Here's the drawing with two shaded views (mm, measured from the low corner). I have some questions. A direction names the side the tool comes from. Round coordinates to 2 decimals unless told otherwise and drop trailing zeros. Loops run counter-clockwise (first coordinate to the right, second up) from the corner with the lowest first, then second, coordinate; pieces in that order, holes last.
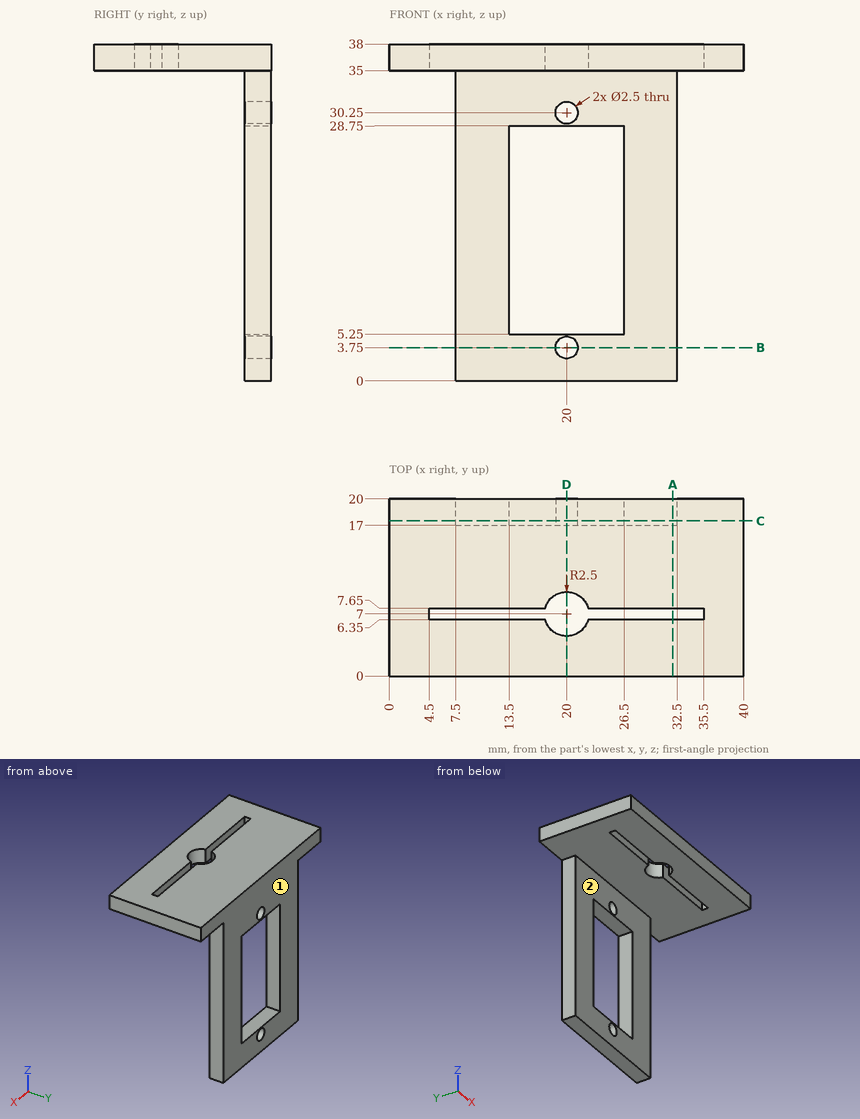
Item 1: If we section it at A-A, the plane x = 32: Please give me the cut outline in (y, z).
Results list:
outline: (0, 35) - (6.35, 35) - (6.35, 38) - (0, 38) - close; (7.65, 35) - (17, 35) - (17, 0) - (20, 0) - (20, 38) - (7.65, 38) - close
Item 2: If we section it at D-D, the plane x = 20: Please give me the cut outline in (y, z).
Results list:
outline: (0, 35) - (4.5, 35) - (4.5, 38) - (0, 38) - close; (9.5, 35) - (17, 35) - (17, 31.5) - (20, 31.5) - (20, 38) - (9.5, 38) - close; (17, 0) - (20, 0) - (20, 2.5) - (17, 2.5) - close; (17, 5) - (20, 5) - (20, 5.25) - (17, 5.25) - close; (17, 28.75) - (20, 28.75) - (20, 29) - (17, 29) - close
Item 3: For the marked faces 1 and 2, which set-ups out of +Z, -Z, +X, -X, +Y, -Y let a thin tool reach every point of the face, with its end or its side?
Results list:
face 1: +Z, -Z, +X, -X, +Y
face 2: -Z, +X, -X, -Y
Item 4: If I drill on line 1 along Z through (x, y) = (20, 17.8); line 2 along X through (y, z) = (19.25, 11.5); line 3 along X through (y, z) = (19.35, 3.75), over which ranges is the centre line in solid material (lowest first)?
Results list:
line 1: z = 0 to 2.5, 5 to 5.25, 28.75 to 29, 31.5 to 38
line 2: x = 7.5 to 13.5, 26.5 to 32.5
line 3: x = 7.5 to 18.75, 21.25 to 32.5
Item 5: If we section it at C-C, the plane y = 17.5: Please give me the cut outline in (x, z), then the cut area to 3 significant figures.
Results list:
outline: (0, 35) - (7.5, 35) - (7.5, 0) - (32.5, 0) - (32.5, 35) - (40, 35) - (40, 38) - (0, 38) - close; hole (13.5, 5.25) - (26.5, 5.25) - (26.5, 28.75) - (13.5, 28.75) - close; hole circle Ø2.5 at (20, 3.75); hole circle Ø2.5 at (20, 30.25)
area: 680 mm2
Item 6: Will these pins go through, and if not, where does the flat tip stop? pin 1 (2.5 mm diameter, centred on y = 18, z = 21, fed in from +X); pin 2 (3 mm diameter, centred on x = 20, z = 3.75, fed in from -Y); pin 3 (3.5 mm diameter, centred on y = 19, z = 18, fed in from -X).
Results list:
pin 1: stops at x = 32.5
pin 2: stops at y = 17
pin 3: stops at x = 7.5
Item 7: If we section it at B-B, the plane z = 3.75: Please give me the cut outline in (x, y).
Results list:
outline: (7.5, 17) - (18.75, 17) - (18.75, 20) - (7.5, 20) - close; (21.25, 17) - (32.5, 17) - (32.5, 20) - (21.25, 20) - close
